Job drawing, mm, ordinate dimensions from the low corner. One solid piece. Coordinates: 2 decimals unless noted, no trailing zeros. Order: outer loops, then holes, each group sorted by start corner. A loop starts at its lowest first (then second) coordinate and runs counter-clockwise, first axis right, second up. Notation, with made-up numbers: (34, 50.25) - (92, 50.25) arc R18 cw to (92, 74.25) - close; hole circle Ø4 at (86, -17.75). An arc over 180 degrees is marked (long way). Return JSON: item names as keys, results as strings.
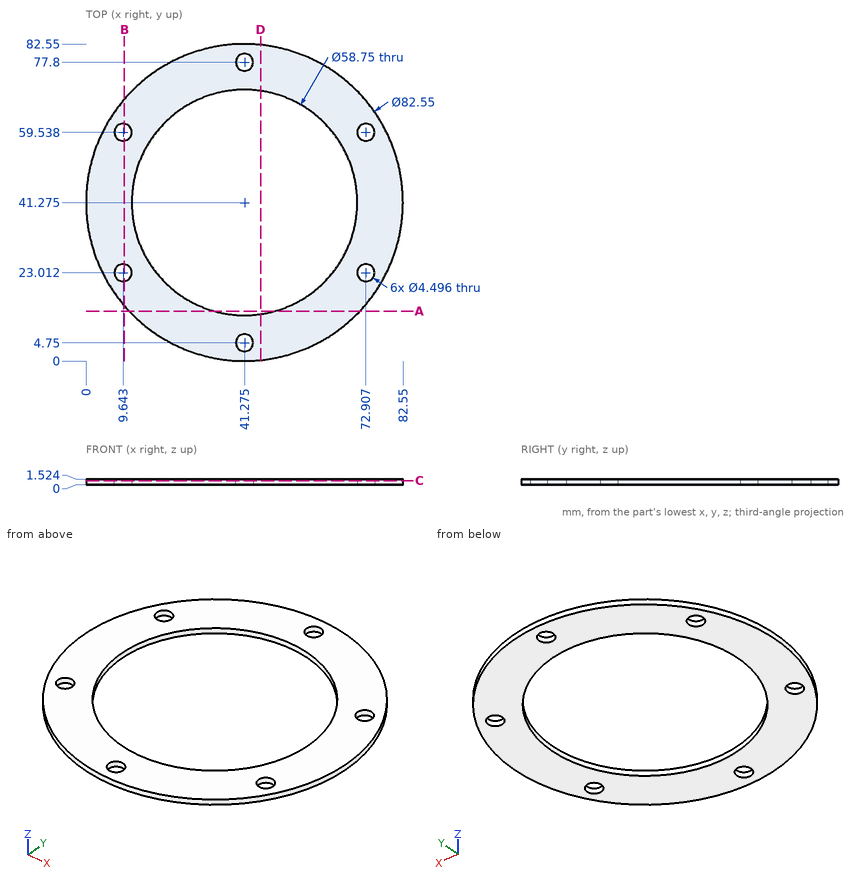
1. Cut at D-D on x = 45.5. Give the cut face in (y, z) (1 decimal).
Check values:
{"outline": "(0.2, 0) - (12.2, 0) - (12.2, 1.5) - (0.2, 1.5) - close; (70.3, 0) - (82.3, 0) - (82.3, 1.5) - (70.3, 1.5) - close"}
2. Cut at B-B on x = 10. Give the cut face in (y, z).
Check values:
{"outline": "(14.34, 0) - (20.79, 0) - (20.79, 1.52) - (14.34, 1.52) - close; (25.23, 0) - (57.32, 0) - (57.32, 1.52) - (25.23, 1.52) - close; (61.76, 0) - (68.21, 0) - (68.21, 1.52) - (61.76, 1.52) - close"}
3. Probe L1, parallel to Y at x = 41.5, z = 1.05; L2, parallel to X at y = 23, z = 0.9 (1 decimal); L3, parallel to Y at x = 42, z = 1.05. List the from-to ranges inside material, lowest first.
Check values:
{"L1": "0 to 2.51, 6.99 to 11.9, 70.65 to 75.56, 80.04 to 82.55", "L2": "4.3 to 7.4, 11.9 to 18.3, 64.3 to 70.7, 75.2 to 78.3", "L3": "0.01 to 2.62, 6.88 to 11.91, 70.64 to 75.67, 79.93 to 82.54"}
4. Cut at A-A on y = 13. Give the cut face in (x, z).
Check values:
{"outline": "(11.21, 0) - (33.31, 0) - (33.31, 1.52) - (11.21, 1.52) - close; (49.24, 0) - (71.34, 0) - (71.34, 1.52) - (49.24, 1.52) - close"}
5. Cut at C-C on z = 1.1. State how many separate pieces and enclosed holes the cut face has, plus the area to 3 significant figures.
Check values:
{"separate pieces": "1", "enclosed holes": "7", "area": "2,550 mm²"}
